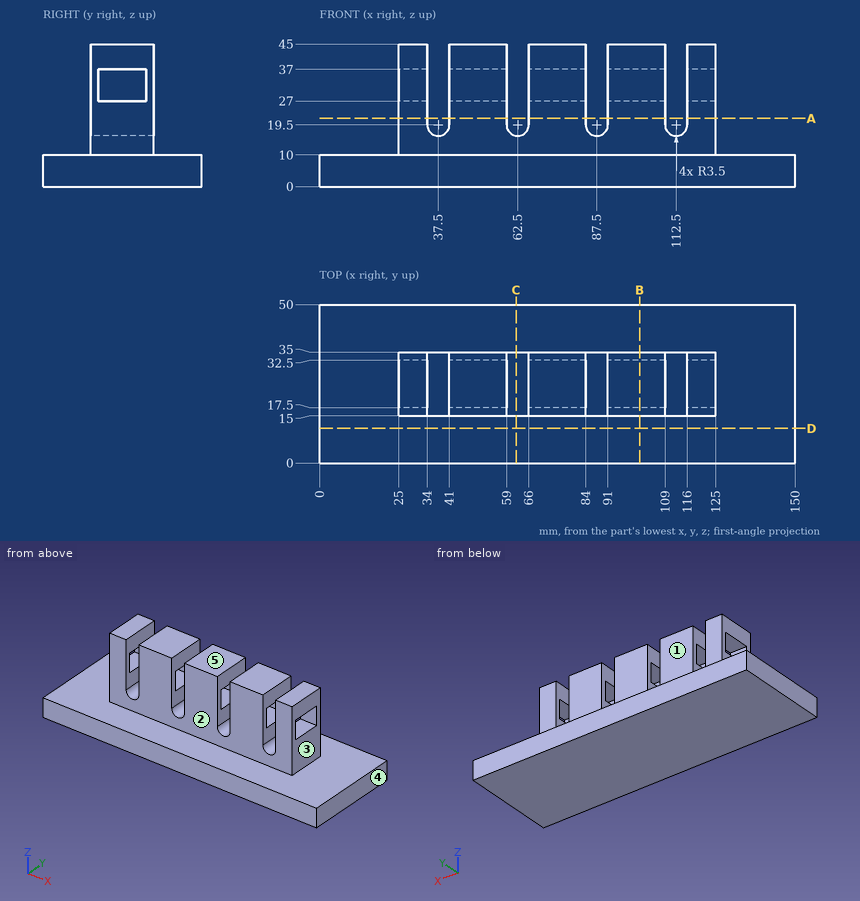
Can you work these out from the drawing? Everything is in mm from the part's minimum corner. A direction names the side the tool comes from. Give positions to 0.01 mm unless a question says otherwise; leave off trailing zeros. Order: outer loops, then holes, each group sorted by start corner. A loop starts at its lowest first (then second) coordinate and runs counter-clockwise, first axis right, second up. Notation, with made-up numbers: M 36.5,17.25 L 93.5,17.25 A28 ccw 93.5,36.25 Z; hole C 19,38 d3. An arc over 180 degrees is marked long. One line per question, with ' | ' between items.
1. I want a section at B-B (x = 101). List the corners of the cut face in (y, z) for me, and give its area (3 significant figures).
Results:
outline: M 0,0 L 50,0 L 50,10 L 35,10 L 35,45 L 15,45 L 15,10 L 0,10 Z; hole M 17.5,27 L 32.5,27 L 32.5,37 L 17.5,37 Z | area: 1,050 mm²
2. For the marked faces 1, 2, 3, 4 and 5, which set-ups out of +Z, -Z, +X, -X, +Y, -Y let a thin tool reach every point of the face, with its end or its side?
Results:
face 1: +Z, +X, -X, +Y | face 2: +Z, +X, -X, -Y | face 3: +Z, +X, +Y, -Y | face 4: +Z, -Z, +X, +Y, -Y | face 5: +Z, +X, -X, +Y, -Y
3. I want a section at C-C (x = 62). List the corners of the cut face in (y, z) for me.
Results:
outline: M 0,0 L 50,0 L 50,10 L 35,10 L 35,16.04 L 15,16.04 L 15,10 L 0,10 Z
4. I'm going to push flat-ended pins straight in: pin 1 (3 mm diameter, centred on x = 74.5, z = 34.5, fed in from +Y); pin 2 (6 mm diameter, centred on y = 29.5, z = 27, fed in from +X); pin 3 (10 mm diameter, centred on y = 24, z = 36, fed in from -X). Where does each tip first touch, or does it pass through?
Results:
pin 1: y = 35 | pin 2: x = 125 | pin 3: x = 25
5. I want a section at D-D (y = 11). List the corners of the cut face in (x, z) for me, and give its area (3 significant figures).
Results:
outline: M 0,0 L 150,0 L 150,10 L 0,10 Z | area: 1,500 mm²
6. I want a section at A-A (z = 21.5). List the corners of the cut face in (x, y) for me, and give its area (3 significant figures).
Results:
outline: M 25,15 L 34,15 L 34,35 L 25,35 Z; M 41,15 L 59,15 L 59,35 L 41,35 Z; M 66,15 L 84,15 L 84,35 L 66,35 Z; M 91,15 L 109,15 L 109,35 L 91,35 Z; M 116,15 L 125,15 L 125,35 L 116,35 Z | area: 1,440 mm²
7. If I drill on line 1 (X direction, y = 30.5, z = 43); line 2 (Y direction, x = 70, z = 32); line 3 (Z direction, x = 128, y = 47.5), over which ranges is the centre line in solid material (lowest first)?
Results:
line 1: 25 to 34, 41 to 59, 66 to 84, 91 to 109, 116 to 125 | line 2: 15 to 17.5, 32.5 to 35 | line 3: 0 to 10
